Autodesk Fusion 360 part; units mm, degrees
sketch "Sketch1" plane through (0, 0, 0) normal (0, 1, 0) x (1, 0, 0)
  circle A0 centre (0, -6.35) radius 5.0165
  dimension "d1" = 10.033
extrude "Extrude1" add sketch "Sketch1" along normal blind 33.02
hole "Hole1" at (0, 55.245, 11.3665) direction (0, 0, -1) diameter 2.54 depth 19.05 tip angle 118
extrude "Extrude2" cut 1 faces at (-0.3721, 0, 4.7198) along direction (0, 1, 0) blind 2.54
sketch "Sketch3" plane through (0, 2.54, 0) normal (0, -1, 0) x (1, 0, 0)
  circle A0 centre (0, 6.35) radius 5.0165
  line L0 (-2.54, 8.89) -> (2.54, 8.89)
  line L1 (2.54, 8.89) -> (2.54, 3.81)
  line L2 (2.54, 3.81) -> (-2.54, 3.81)
  line L3 (-2.54, 3.81) -> (-2.54, 8.89)
extrude "Extrude3" add sketch "Sketch3" along normal blind 2.54 contours L0 L1 L2 L3
extrude "Extrude4" add 1 faces at (0.8467, 0.8467, 8.89) along direction (0, 0, 1) blind 3.302
extrude "Extrude5" add 1 faces at (2.54, 0.8467, 8.8926) along direction (1, 0, 0) blind 3.302
extrude "Extrude6" add 1 faces at (2.5426, 0.8467, 3.81) along direction (0, 0, -1) blind 3.302
extrude "Extrude7" add 1 faces at (-2.54, 0.8467, 4.908) along direction (-1, 0, 0) blind 3.302
fillet "Fillet1" radius 5.842 4 edges at (-5.842, 1.27, 12.192) (5.842, 1.27, 12.192) (5.842, 1.27, 0.508) (-5.842, 1.27, 0.508)
hole "Hole2" at (0, 30.48, 11.3665) direction (0, 0, -1) diameter 2.54 depth 23.622 tip angle 118
Build history of the part. All positions in model axes, mm. A direction names the side the tool comes from. Give positions to 0.01 mm unless a question says otherwise; leave off trailing zeros. Order: outer loops, then holes, each group sorted by start corner. A loop starts at its lowest first (then second) coordinate and runs counter-clockwise, first axis right, second up. Notation, with made-up numbers: M 70,47.5 L 98,47.5 A19 cw 98,82.5 Z; hole C 64.25,51.25 d5. An arc over 180 degrees is marked long. Put each result on its own line as item: value.
Item 1: Two-plate mould, pull along Y, no slides. Class faces 1 (the flat face through (0, 0, 6)), 2 (the flat face through (5, 2.54, 5)), 3 (the cylindrical face through (-4.086, 1.252, 10.526)), 4 (the cylindrical face through (-0.38, 29.27, 6.28)): +Y half, -Y half, draft (parallel to the pull), parting line (faces both ways), or undercut.
From the geometry:
face 1: -Y half
face 2: +Y half
face 3: draft
face 4: undercut
Item 2: Slice it at B-B, the plane z = 8.25. Write the cut outline in (x, y), plus the area to 3 significant figures.
From the geometry:
outline: M -5.52,0 L 5.52,0 L 5.52,2.54 L 4.64,2.54 L 4.64,33.02 L -4.64,33.02 L -4.64,2.54 L -5.52,2.54 Z; hole C 0,30.48 d2.54
area: 306 mm2
Item 3: Probe line 1 (Y direction, x = 0, z = 9.75); line 2 (X direction, y = 30.48, z = 5.5); line 3 (X direction, y = 23, z = 6.5). List the from-to ranges inside material, lowest first. Write a range as [from, to].
From the geometry:
line 1: y = [0, 29.21], [31.75, 33.02]
line 2: x = [-4.94, -1.27], [1.27, 4.94]
line 3: x = [-5.01, 5.01]
Item 4: Slice it at D-D, the plane x = -3. Write the cut outline in (y, z).
From the geometry:
outline: M 0,1.34 L 2.54,1.34 L 2.54,2.33 L 33.02,2.33 L 33.02,10.37 L 2.54,10.37 L 2.54,11.36 L 0,11.36 Z
Item 5: 3-axis set-ups, long thin cutter, end or side, ignore diameter. For faces 5 (the cylindrical face through (-4.176, 1.252, 2.264)), 6 (the cylindrical face through (4.785, 17.567, 7.857)): which of +Z, -Z, +X, -X, +Y, -Y reach the whole face in a straight line?
From the geometry:
face 5: -Z, -X, +Y, -Y
face 6: +Y
Item 6: Slice it at C-C, the plane y = 30.48. Write the cut outline in (x, z).
From the geometry:
outline: M -1.27,1.5 L -1.27,11.2 A5.02 ccw Z; M 1.27,1.5 A5.02 ccw 1.27,11.2 Z
Item 7: Flat gauge pins, fed straight in: pin 1 Ø1 at (x, y) = (-1, 13) entering from -Z; pin 2 Ø1.5 at (x, y) = (2, 18) entering from +Z; pin 3 Ø4 at (y, z) = (19, 5) entering from +X. Where does each tip first touch, or does it go through?
From the geometry:
pin 1: stops at z = 1.36
pin 2: stops at z = 11.21
pin 3: stops at x = 5.02
